from build123d import *

# Parameters (mm, degrees)
SKETCH1_W           = 30
SKETCH1_H           = 16.7
SKETCH1_W_2         = 20
SKETCH1_H_2         = 6.7
BOSS_EXTRUDE1_DEPTH = 25
SKETCH1_3_W         = 20
SKETCH1_3_H         = 1
BOSS_EXTRUDE2_DEPTH = 13
SKETCH2_W           = 15
SKETCH2_H           = 25
BOSS_EXTRUDE3_DEPTH = 16.7
CHAMFER1_SIZE       = 2
CHAMFER2_SIZE       = 2


with BuildPart() as part:
    # Sketch1 → Boss-Extrude1 (new body)
    with BuildSketch(Plane(origin=(0, 0, 0), x_dir=(1, 0, 0), z_dir=(0, 1, 0))):
        with Locations((15, 8.35)):
            Rectangle(SKETCH1_W, SKETCH1_H)
        with Locations((15, 8.35)):
            Rectangle(SKETCH1_W_2, SKETCH1_H_2, mode=Mode.SUBTRACT)
    extrude(amount=BOSS_EXTRUDE1_DEPTH)

    # Sketch1<3> → Boss-Extrude2 (add)
    with BuildSketch(Plane(origin=(0, 0, 0), x_dir=(1, 0, 0), z_dir=(0, 1, 0))):
        with Locations((15, 11.2)):
            Rectangle(SKETCH1_3_W, SKETCH1_3_H)
        with Locations((15, 5.5)):
            Rectangle(SKETCH1_3_W, SKETCH1_3_H)
    extrude(amount=BOSS_EXTRUDE2_DEPTH)

    # Sketch2 → Boss-Extrude3 (add, through all)
    # profile 1 of 2: a face of its own
    with BuildSketch(Plane(origin=(0, 0, -16.7), x_dir=(-1, 0, 0), z_dir=(0, 0, -1))):
        with Locations((-37.5, 12.5)):
            Rectangle(SKETCH2_W, SKETCH2_H)
        with BuildLine():
            Line((-40.25, 5.75), (-40.25, 19.25))
            ThreePointArc((-40.25, 19.25), (-37.5, 22), (-34.75, 19.25))
            Line((-34.75, 19.25), (-34.75, 5.75))
            ThreePointArc((-34.75, 5.75), (-37.5, 3), (-40.25, 5.75))
        make_face(mode=Mode.SUBTRACT)
    # profile 2 of 2: a face of its own
    with BuildSketch(Plane(origin=(0, 0, -16.7), x_dir=(-1, 0, 0), z_dir=(0, 0, -1))):
        with Locations((7.5, 12.5)):
            Rectangle(SKETCH2_W, SKETCH2_H)
        with BuildLine():
            Line((10.25, 5.75), (10.25, 19.25))
            ThreePointArc((10.25, 19.25), (7.5, 22), (4.75, 19.25))
            Line((4.75, 19.25), (4.75, 5.75))
            ThreePointArc((4.75, 5.75), (7.5, 3), (10.25, 5.75))
        make_face(mode=Mode.SUBTRACT)
    extrude(amount=-BOSS_EXTRUDE3_DEPTH)

    # Chamfer1
    chamfer1_edges = [part.edges().sort_by_distance(p)[0] for p in [
        (15, 25, -16.7),
        (45, 25, -8.35),
        (-15, 25, -8.35),
        (15, 25, 0),
    ]]
    chamfer(chamfer1_edges, length=CHAMFER1_SIZE)

    # Chamfer2
    chamfer2_edges = [part.edges().sort_by_distance(p)[0] for p in [
        (45, 11.5, -16.7),
        (45, 11.5, 0),
        (15, 0, -16.7),
        (15, 0, 0),
        (25, 0, -8.35),
        (5, 0, -8.35),
        (15, 0, -10.7),
        (15, 0, -6),
        (45, 0, -8.35),
        (-15, 11.5, 0),
        (-15, 0, -8.35),
        (-15, 11.5, -16.7),
    ]]
    chamfer(chamfer2_edges, length=CHAMFER2_SIZE)


solid = part.part
The model under review builds one solid part; all positions refer to its coordinate system, in mm. A direction names the side the tool comes from. Round coordinates to 2 decimals unless told otherwise and drop trailing zeros. Loops run counter-clockwise (first coordinate to the right, second up) from the corner with the lowest first, then second, coordinate; pieces in that order, holes last. Notation, with made-up numbers: (42, 19) -> (51, 19) arc R16 cw to (51, 47) -> close; hole circle Ø7 at (43.25, 74). An arc over 180 degrees is marked (long way). Answer as CSV lines item,"result".
1) Add section C-C on z = -7. Write out the cut boundary in (x, y).
Geometry results:
outline,"(-15, 2) -> (-13, 0) -> (3, 0) -> (5, 2) -> (5, 25) -> (-13, 25) -> (-15, 23) -> close; (25, 2) -> (27, 0) -> (43, 0) -> (45, 2) -> (45, 23) -> (43, 25) -> (25, 25) -> close; hole (-10.25, 5.75) arc R2.75 ccw to (-4.75, 5.75) -> (-4.75, 19.25) arc R2.75 ccw to (-10.25, 19.25) -> close; hole (34.75, 5.75) arc R2.75 ccw to (40.25, 5.75) -> (40.25, 19.25) arc R2.75 ccw to (34.75, 19.25) -> close"
2) Add section D-D on y = 14. Write out the cut boundary in (x, z), plus the area to 3 significant figures.
Geometry results:
outline,"(-15, -14.7) -> (-13, -16.7) -> (-10.25, -16.7) -> (-10.25, 0) -> (-13, 0) -> (-15, -2) -> close; (-4.75, -16.7) -> (34.75, -16.7) -> (34.75, 0) -> (-4.75, 0) -> close; (40.25, -16.7) -> (43, -16.7) -> (45, -14.7) -> (45, -2) -> (43, 0) -> (40.25, 0) -> close; hole (5, -11.7) -> (25, -11.7) -> (25, -5) -> (5, -5) -> close"
area,"676 mm²"
3) To check wall thickness, follow line 1 along X through (y, z) = (5.75, -4); line 2 along X through (y, z) = (16.5, -8.75); line 3 along X through (y, z) = (21, -2.75). State the ranges of each line that lie inside material, in increasing order. Write a range as from..to.
Geometry results:
line 1,"x = -15..-10.25, -4.75..34.75, 40.25..45"
line 2,"x = -15..-10.25, -4.75..5, 25..34.75, 40.25..45"
line 3,"x = -15..-9.62, -5.38..35.38, 39.62..45"
4) For P1, Ø0.5, axis at x = 18, z = -5.5, coming from the +Y side; P2, Ø3, axis at x = 19.5, z = -7, coming from the -Y side, all flat-tipped, find the tip position at first contact; note any pin that passes through.
Geometry results:
P1,"stops at y = 13"
P2,"stops at y = 1.5"
5) Add section A-A on y = 6.5. Write out the cut boundary in (x, z).
Geometry results:
outline,"(-15, -14.7) -> (-13, -16.7) -> (-10.25, -16.7) -> (-10.25, 0) -> (-13, 0) -> (-15, -2) -> close; (-4.75, -16.7) -> (34.75, -16.7) -> (34.75, 0) -> (-4.75, 0) -> close; (40.25, -16.7) -> (43, -16.7) -> (45, -14.7) -> (45, -2) -> (43, 0) -> (40.25, 0) -> close; hole (5, -10.7) -> (25, -10.7) -> (25, -6) -> (5, -6) -> close"
6) Tool access review of faces 1 (the face through (25, 13, -8)), 2 (the face through (-7.4, 3, -8.5)), 3 (the face through (14.8, 1, -11.7)): name each direction out of +Z, -Z, +X, -X, +Y, -Y from which nothing blocks a thin tool from reaching the whole face with its end or side.
Geometry results:
face 1,"+Y"
face 2,"+Z, -Z"
face 3,"-Y"
7) Add section B-B on x = 19.5. Write out the cut boundary in (y, z).
Geometry results:
outline,"(0, -14.7) -> (2, -16.7) -> (23, -16.7) -> (25, -14.7) -> (25, -11.7) -> (13, -11.7) -> (13, -10.7) -> (2, -10.7) -> (0, -12.7) -> close; (0, -4) -> (2, -6) -> (13, -6) -> (13, -5) -> (25, -5) -> (25, -2) -> (23, 0) -> (2, 0) -> (0, -2) -> close"
8) Draft analysis for pull direction Z (two halves, no side actions). For faces 4 (the face through (15, 7, -10.7)), 5 (the face through (-13.8, 1.4, -15.3)), 6 (the face through (40.25, 12, -8)), 7 (the face through (15, 13, 0)), state which applies: pulls with the +Z half, pulls with the -Z half, needs draft (parallel to the pull), parting line crosses it, or undercut.
Geometry results:
face 4,"undercut"
face 5,"pulls with the -Z half"
face 6,"needs draft"
face 7,"pulls with the +Z half"
